Work out the finished part from the listing and answer in its coordinate system (mm). Give positions to 0.01 mm unless a question says otherwise; leave off trailing zeros. Loops run counter-clockwise (first coordinate to the right, second up) from the corner with the lowest first, then second, coordinate; pieces in that order, holes last.
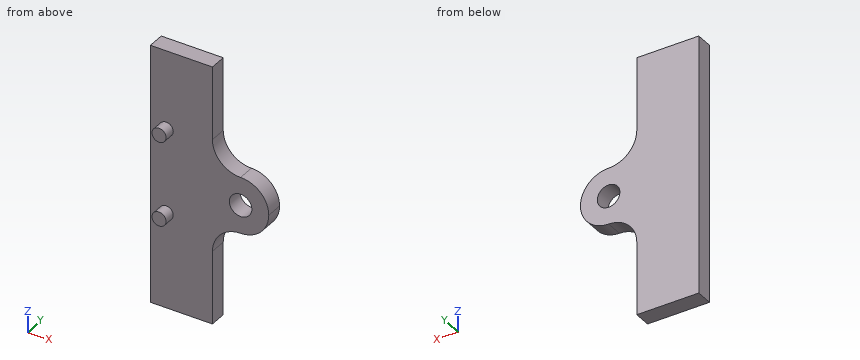
```python
from build123d import *

# Parameters (mm, degrees)
SKETCH1_W           = 9
SKETCH1_H           = 46
BOSS_EXTRUDE1_DEPTH = 3
SKETCH2_R           = 1.25
BOSS_EXTRUDE2_DEPTH = 5
SKETCH3_W           = 46
SKETCH3_H           = 3
BOSS_EXTRUDE3_DEPTH = 2
SKETCH4_W           = 10
SKETCH4_H           = 3
BOSS_EXTRUDE4_DEPTH = 10
SKETCH5_R           = 2
CUT_EXTRUDE1_DEPTH  = 10
FILLET1_R           = 5
FILLET2_R           = 5


with BuildPart() as part:
    # Sketch1 → Boss-Extrude1 (new body)
    with BuildSketch(Plane(origin=(0, 0, 0), x_dir=(1, 0, 0), z_dir=(0, 1, 0))):
        Rectangle(SKETCH1_W, SKETCH1_H)
    extrude(amount=BOSS_EXTRUDE1_DEPTH)

    # Sketch2 → Boss-Extrude2 (add)
    with BuildSketch(Plane(origin=(0, 3, 0), x_dir=(1, 0, 0), z_dir=(0, 1, 0))):
        with Locations(Location((-1.7, -9, 0), (0, 0, 270))):
            Circle(SKETCH2_R)
        with Locations(Location((-1.7, 6, 0), (0, 0, 270))):
            Circle(SKETCH2_R)
    extrude(amount=-BOSS_EXTRUDE2_DEPTH)

    # Sketch3 → Boss-Extrude3 (add)
    with BuildSketch(Plane(origin=(4.5, 0, 0), x_dir=(0, 0, -1), z_dir=(1, 0, 0))):
        with Locations((0, 1.5)):
            Rectangle(SKETCH3_W, SKETCH3_H)
    extrude(amount=BOSS_EXTRUDE3_DEPTH)

    # Sketch4 → Boss-Extrude4 (add)
    with BuildSketch(Plane(origin=(6.5, 0, 0), x_dir=(0, 0, -1), z_dir=(1, 0, 0))):
        with Locations((0, 1.5)):
            Rectangle(SKETCH4_W, SKETCH4_H)
    extrude(amount=BOSS_EXTRUDE4_DEPTH)

    # Sketch5 → Cut-Extrude1 (cut)
    with BuildSketch(Plane(origin=(0, 3, 0), x_dir=(1, 0, 0), z_dir=(0, 1, 0))):
        with Locations(Location((11.5, 0, 0), (0, 0, 270))):
            Circle(SKETCH5_R)
    extrude(amount=-CUT_EXTRUDE1_DEPTH, mode=Mode.SUBTRACT)

    # Fillet1
    fillet1_edges = [part.edges().sort_by_distance(p)[0] for p in [
        (16.5, 1.5, 5),
        (16.5, 1.5, -5),
    ]]
    fillet(fillet1_edges, radius=FILLET1_R - 0.0001)  # a hair under: the kernel refuses the full size

    # Fillet2
    fillet2_edges = [part.edges().sort_by_distance(p)[0] for p in [
        (6.5, 1.5, -5),
        (6.5, 1.5, 5),
    ]]
    fillet(fillet2_edges, radius=FILLET2_R)


solid = part.part
```
Q1. Section D-D on x = 13 is taken. Give the vertices of the cut face in (y, z), plus the area to 3 significant figures.
Q2. Section A-A on x = -1.7 is taken. Give the vertices of the cut face in (y, z), plus the area to 3 significant figures.
Q3. Consider line 1 along X through (y, z) = (1.15, 0); line 2 along X through (y, z) = (0.3, 21); line 3 along Y through (x, z) = (-3, 20). Determine where each line is inside the solid, lowest interval first.
Q4. Section C-C on z = 9 is taken. Give the vertices of the cut face in (x, y).
Q5. Given pin 1 (1.5 mm diameter, centred on y = 1, z = -17, fed in from +X); pin 2 (6.5 mm diameter, centred on x = 3.5, z = -11, fed in from -Y), each flat-ended and moving along its own axis, determine where each tip first touches the part or whether it passes through.
Check result:
1. outline: (0, -4.77) - (3, -4.77) - (3, -1.32) - (0, -1.32) - close; (0, 1.32) - (3, 1.32) - (3, 4.77) - (0, 4.77) - close
1. area: 20.7 mm2
2. outline: (-2, -7.25) - (0, -7.25) - (0, -23) - (3, -23) - (3, 23) - (0, 23) - (0, 10.25) - (-2, 10.25) - (-2, 7.75) - (0, 7.75) - (0, -4.75) - (-2, -4.75) - close
2. area: 148 mm2
3. line 1: x = -4.5 to 9.5, 13.5 to 16.5
3. line 2: x = -4.5 to 6.5
3. line 3: y = 0 to 3
4. outline: (-4.5, 0) - (-2.95, 0) - (-2.95, -2) - (-0.45, -2) - (-0.45, 0) - (6.6, 0) - (6.6, 3) - (-4.5, 3) - close
5. pin 1: stops at x = 6.5
5. pin 2: stops at y = 0
